```python
from build123d import *

# Parameters (mm, degrees)
SKETCH1_R                                      = 76.2
BILLET_DEPTH                                   = 50.8
SKETCH3_R                                      = 19.05
LOX_PLATE_DEPTH                                = 13.97
SKETCH5_R                                      = 13.97
LOX_DOME_DEPTH                                 = 20.32
SKETCH7_R                                      = 76.2
TOP_MILL_DEPTH                                 = 12.7
F_1_4_BOLT_HOLE_REACH                          = 116.3
SKETCH11_R                                     = 3.175
BOLT_PATTERN_COUNT                             = 8
SKETCH12_R                                     = 60.96
KEROSENE_PLATE_DEPTH                           = 10.16
KEROSENE_INLET_3_8_NPT_TAPPED_HOLE1_AT_2_COUNT = 2
KEROSENE_INLET_3_8_NPT_TAPPED_HOLE1_AT_2_PITCH = 63.5
MANIFOLD_HOLE_REACH                            = 121.137
SKETCH14_R                                     = 3.175
SKETCH15_R                                     = 8.89
SKETCH15_R_2                                   = 7.62
MANIFOLD_SEAL_DEPTH                            = 1.27
SKETCH26_R                                     = 17.78
SKETCH26_R_2                                   = 16.51
LOX_PLATE_O_RING_DEPTH                         = 1.27


with BuildPart() as part:
    # Sketch1 → Billet (new body)
    with BuildSketch(Plane(origin=(0, 0, 0), x_dir=(1, 0, 0), z_dir=(0, 1, 0))):
        with Locations(Location((0, 0, 0), (0, 0, 270))):
            Circle(SKETCH1_R)
    extrude(amount=-BILLET_DEPTH)

    # Sketch3 → Lox Plate (cut)
    with BuildSketch(Plane(origin=(0, -50.8, 0), x_dir=(1, 0, 0), z_dir=(0, 1, 0))):
        with Locations(Location((0, 0, 0), (0, 0, 270))):
            Circle(SKETCH3_R)
    extrude(amount=LOX_PLATE_DEPTH, mode=Mode.SUBTRACT)

    # Sketch5 → Lox Dome (cut)
    with BuildSketch(Plane(origin=(0, -50.8, 0), x_dir=(1, 0, 0), z_dir=(0, 1, 0))):
        with Locations(Location((0, 0, 0), (0, 0, 270))):
            Circle(SKETCH5_R)
    extrude(amount=LOX_DOME_DEPTH, mode=Mode.SUBTRACT)

    # Sketch7 → Top Mill (cut)
    with BuildSketch(Plane(origin=(0, 0, 0), x_dir=(1, 0, 0), z_dir=(0, 1, 0))):
        with Locations(Location((0, 0, 0), (0, 0, 270))):
            Circle(SKETCH7_R)
    extrude(amount=-TOP_MILL_DEPTH, mode=Mode.SUBTRACT)

    # Sketch11 → 1_4_ Bolt Hole (cut, up to next)
    with BuildSketch(Plane(origin=(0, -50.8, 0), x_dir=(1, 0, 0), z_dir=(0, 1, 0)), mode=Mode.PRIVATE) as f_1_4_bolt_hole_sk1:
        with Locations(Location((0, 68.58, 0), (0, 0, 270))):
            Circle(SKETCH11_R)
    f_1_4_bolt_hole_tool1 = extrude(f_1_4_bolt_hole_sk1.sketch, amount=F_1_4_BOLT_HOLE_REACH, mode=Mode.PRIVATE) & part.part
    f_1_4_bolt_hole = f_1_4_bolt_hole_tool1.solids().sort_by_distance((0, -50.8, -68.58))[0]
    add(f_1_4_bolt_hole, mode=Mode.SUBTRACT)

    # Bolt Pattern: 1_4_ Bolt Hole ×8 about axis
    bolt_pattern_axis = Axis((0, 0, 0), (0, 1, 0))
    for i in range(1, BOLT_PATTERN_COUNT):
        add(f_1_4_bolt_hole.rotate(bolt_pattern_axis, i * 360 / BOLT_PATTERN_COUNT), mode=Mode.SUBTRACT)

    # Sketch12 → Kerosene Plate (cut)
    with BuildSketch(Plane(origin=(0, -50.8, 0), x_dir=(1, 0, 0), z_dir=(0, 1, 0))):
        with Locations(Location((0, 0, 0), (0, 0, 270))):
            Circle(SKETCH12_R)
    extrude(amount=KEROSENE_PLATE_DEPTH, mode=Mode.SUBTRACT)

    # Sketch21 → Lox Inlet-1_2 NPT Tapped Hole3 (revolve, cut)
    with BuildSketch(Plane(origin=(0, -12.7, 5.08), x_dir=(0, 0, 1), z_dir=(1, 0, 0))):
        Polygon((0, 0), (0, 38.1), (8.9281, 38.1), (8.9281, 13.462), (10.261665792, 13.462), (10.6647361, 0), align=None)
    revolve(axis=Axis((0, -6.35, 5.08), (0, -1, 0)), mode=Mode.SUBTRACT)

    # Sketch25 → Kerosene Inlet-3_8 NPT Tapped Hole1 (revolve, cut)
    with BuildSketch(Plane(origin=(-31.75, -12.7, 0), x_dir=(0, 0, 1), z_dir=(1, 0, 0))):
        Polygon((0, 0), (0, 38.1), (7.1374, 38.1), (7.1374, 10.414), (8.263205494, 10.414), (8.5750146, 0), align=None)
    kerosene_inlet_3_8_npt_tapped_hole1 = revolve(axis=Axis((-31.75, -6.35, 0), (0, -1, 0)), mode=Mode.SUBTRACT)

    # Kerosene Inlet-3_8 NPT Tapped Hole1 at 2: Kerosene Inlet-3_8 NPT Tapped Hole1 ×2
    with Locations(*[(i * KEROSENE_INLET_3_8_NPT_TAPPED_HOLE1_AT_2_PITCH, 0, 0) for i in range(1, KEROSENE_INLET_3_8_NPT_TAPPED_HOLE1_AT_2_COUNT)]):
        add(kerosene_inlet_3_8_npt_tapped_hole1, mode=Mode.SUBTRACT)

    # Sketch14 → Manifold hole (cut, up to next)
    with BuildSketch(Plane(origin=(0, 0, 0), x_dir=(1, 0, 0), z_dir=(0, 1, 0)), mode=Mode.PRIVATE) as manifold_hole_sk1:
        with Locations(Location((0, 33.02, 0), (0, 0, 270))):
            Circle(SKETCH14_R)
    manifold_hole_tool1 = extrude(manifold_hole_sk1.sketch, amount=-MANIFOLD_HOLE_REACH, mode=Mode.PRIVATE) & part.part
    add(manifold_hole_tool1.solids().sort_by_distance((0, 0, -33.02))[0], mode=Mode.SUBTRACT)

    # Sketch15 → Manifold seal (cut)
    with BuildSketch(Plane(origin=(0, -40.64, 0), x_dir=(1, 0, 0), z_dir=(0, 1, 0))):
        with Locations(Location((0, 33.02, 0), (0, 0, 270))):
            Circle(SKETCH15_R)
        with Locations(Location((0, 33.02, 0), (0, 0, 270))):
            Circle(SKETCH15_R_2, mode=Mode.SUBTRACT)
    extrude(amount=MANIFOLD_SEAL_DEPTH, mode=Mode.SUBTRACT)

    # Sketch26 → Lox Plate O Ring (cut)
    with BuildSketch(Plane.XZ.offset(36.83)):
        with Locations(Location((0, 0, 0), (0, 0, 270))):
            Circle(SKETCH26_R)
        with Locations(Location((0, 0, 0), (0, 0, 270))):
            Circle(SKETCH26_R_2, mode=Mode.SUBTRACT)
    extrude(amount=-LOX_PLATE_O_RING_DEPTH, mode=Mode.SUBTRACT)


solid = part.part
```
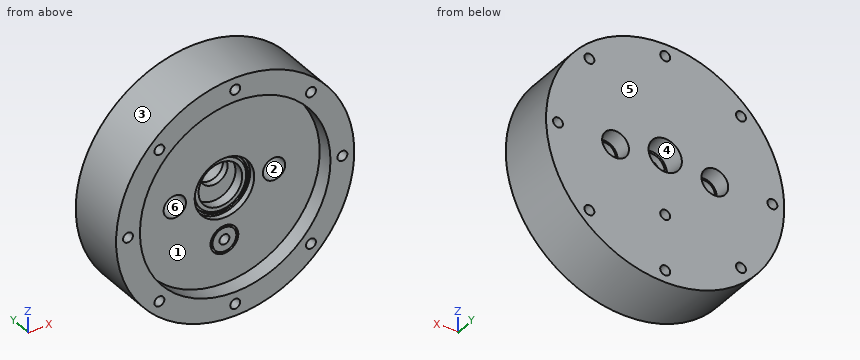
Here's how the part is built. I have some questions about the finished solid (model axes, mm). Face numbers are marked on the shaded views. A direction names the side the tool comes from. Coordinates: 2 decimals unless noted, no trailing zeros. Order: outer loops, then holes, each group sorted by start corner. A loop starts at its lowest first (then second) coordinate and runs counter-clockwise, first axis right, second up.
Item 1: If we section it at A-A, the plane z = 68.58: List the corners of the cut face in (x, y) for me (3 decimals).
Response values:
outline: (-33.215, -50.8) - (-3.175, -50.8) - (-3.175, -12.7) - (-33.215, -12.7) - close; (3.175, -50.8) - (33.215, -50.8) - (33.215, -12.7) - (3.175, -12.7) - close
Item 2: If we section it at B-B, the plane x = -31.75: List the corners of the cut face in (y, z) for me, then the cut area to 3 significant figures.
Response values:
outline: (-50.8, -69.27) - (-12.7, -69.27) - (-12.7, -8.58) - (-23.11, -8.26) - (-23.11, -7.14) - (-40.64, -7.14) - (-40.64, -52.04) - (-50.8, -52.04) - close; (-50.8, 52.04) - (-40.64, 52.04) - (-40.64, 7.14) - (-23.11, 7.14) - (-23.11, 8.26) - (-12.7, 8.58) - (-12.7, 69.27) - (-50.8, 69.27) - close
area: 3,800 mm2
Item 3: I'm going to push flat-ended pins straight in: pin 1 Ø2 at (x, y) = (-56, -35.5) entering from -Z; pin 2 Ø8.5 at (x, z) = (30, 4) entering from +Y; pin 3 Ø1 at (y, z) = (-41.5, -17) entering from +X; pin 4 Ø5 at (y, z) = (-17.5, 0.5) entering from -X. Where does each tip first touch, or does it pass through?
Response values:
pin 1: stops at z = -52.74
pin 2: stops at y = -12.7
pin 3: stops at x = 74.39
pin 4: stops at x = -76.2
Item 4: I need wall thicknesses on probe 1 along Z at (x, y) = (-50.5, -44); probe 2 along X at (y, z) = (-16, 49); probe 3 along Z at (x, y) = (-48.5, -32). Which ranges of each line are inside material? Lowest first, please.
Response values:
probe 1: z = -57.06 to -50.95, -46.03 to -34.14, 34.14 to 46.03, 50.95 to 57.06
probe 2: x = -58.36 to -51.63, -45.36 to 45.36, 51.63 to 58.36
probe 3: z = -58.77 to -51.67, -45.32 to 45.32, 51.67 to 58.77
Item 5: Which directions (+Z, -Z, +X, -X, +Y, -Y) give clear straight access to the entire face, cutting with the end or side of a thin tool? Please do the marked faces 1 and 2.
Response values:
face 1: -Y
face 2: +Y, -Y
Item 6: If we section it at C-C, the plane y = -19.5: Give the number of separate pieces and of enclosed holes in the cut face, then the cut area to 3 significant figures.
Response values:
separate pieces: 1
enclosed holes: 12
area: 17,200 mm2
Item 7: If we section it at D-D, the plane z = 34.5: List the corners of the cut face in (x, y) for me.
Response values:
outline: (-67.94, -50.8) - (-50.26, -50.8) - (-50.26, -40.64) - (50.26, -40.64) - (50.26, -50.8) - (67.94, -50.8) - (67.94, -12.7) - (-67.94, -12.7) - close
Item 8: Thinking about a two-plate mould opening in Z: for the marked faces 3, 4, 5 and 6, which applies, pulls with the +Z half, pulls with the -Z half, needs draft (parallel to the pull), parting line crosses it, or undercut?
Response values:
face 3: parting line crosses it
face 4: undercut
face 5: needs draft
face 6: undercut
